from build123d import *

# Parameters (mm, degrees)
SKETCH11_R                        = 5.5626
BASE_FLANGE1_DEPTH                = 2.286
CSK_FOR_M4_FH_MODIFIED_AT_2_COUNT = 2
CSK_FOR_M4_FH_MODIFIED_AT_2_PITCH = 67.76892481
CSK_FOR_M4_FH_MODIFIED_AT_3_COUNT = 2
CSK_FOR_M4_FH_MODIFIED_AT_3_PITCH = 86
CSK_FOR_M4_FH_MODIFIED_AT_4_COUNT = 2
CSK_FOR_M4_FH_MODIFIED_AT_4_PITCH = 52.946886878
CUT_EXTRUDE1_DEPTH                = 82.450069543
FILLET1_R                         = 6.35


# Sheet-metal steps are written as plain solids
with BuildPart() as part:
    # Sketch11 → Base-Flange1 (new body)
    with BuildSketch(Plane.XY):
        Polygon((-49.2252, 40.4876), (-49.2252, -40.4876), (37.337994573, -40.4876), (70.6374, 17.188662062), (70.6374, 40.4876), align=None)
        with Locations((57.15, 27.0002)):
            Circle(SKETCH11_R, mode=Mode.SUBTRACT)
    extrude(amount=-BASE_FLANGE1_DEPTH)

    # Sketch15 → CSK for M4 FH Modified (revolve, cut)
    with BuildSketch(Plane(origin=(36.062834422, 23.419478506, -2.286), x_dir=(0, 1, 0), z_dir=(1, 0, 0))):
        Polygon((0, 0), (0, 2.286), (3.175, 2.286), (3.175, 1.524), (4.699, 0), align=None)
    csk_for_m4_fh_modified = revolve(axis=Axis((36.062834422, 23.419478506, -8.636), (0, 0, 1)), mode=Mode.SUBTRACT)

    # CSK for M4 FH Modified at 2: CSK for M4 FH Modified ×2
    with Locations(*[Vector(-0.9961946980917455, 0.08715574274765803, 0) * (i * CSK_FOR_M4_FH_MODIFIED_AT_2_PITCH) for i in range(1, CSK_FOR_M4_FH_MODIFIED_AT_2_COUNT)]):
        add(csk_for_m4_fh_modified, mode=Mode.SUBTRACT)

    # CSK for M4 FH Modified at 3: CSK for M4 FH Modified ×2
    with Locations(*[Vector(-0.838670567945423, -0.5446390350150286, 0) * (i * CSK_FOR_M4_FH_MODIFIED_AT_3_PITCH) for i in range(1, CSK_FOR_M4_FH_MODIFIED_AT_3_COUNT)]):
        add(csk_for_m4_fh_modified, mode=Mode.SUBTRACT)

    # CSK for M4 FH Modified at 4: CSK for M4 FH Modified ×2
    with Locations(*[Vector(-0.08715574274765796, -0.9961946980917455, 0) * (i * CSK_FOR_M4_FH_MODIFIED_AT_4_PITCH) for i in range(1, CSK_FOR_M4_FH_MODIFIED_AT_4_COUNT)]):
        add(csk_for_m4_fh_modified, mode=Mode.SUBTRACT)

    # Sketch17 → Cut-Extrude1 (cut, through all)
    with BuildSketch(Plane.XY):
        Polygon((-34.546735645, 48.1076), (-56.8452, 0.288388874), (-56.8452, 48.1076), align=None)
    extrude(amount=-CUT_EXTRUDE1_DEPTH, mode=Mode.SUBTRACT)

    # Fillet1
    fillet1_edges = [part.edges().sort_by_distance(p)[0] for p in [
        (-49.2252, 16.629531608, -1.143),
        (-38.1, 40.4876, -1.143),
        (37.337994573, -40.4876, -1.143),
        (-49.2252, -40.4876, -1.143),
        (70.6374, 40.4876, -1.143),
    ]]
    fillet(fillet1_edges, radius=FILLET1_R)


solid = part.part
Work out the finished part from the listing and answer in its coordinate system (mm). Round coordinates to 2 decimals unless told otherwise and drop trailing zeros. Loops run counter-clockwise (first coordinate to the right, second up) from the corner with the lowest first, then second, coordinate; pieces in that order, holes last. Notation, with made-up numbers: M 42,60.5 L 71,60.5 A7 ccw 71,68.5 Z; hole C 25,43.5 d11. An arc over 180 degrees is marked long. One line per question, with ' | ' between items. Start each with the question number.
(1) A cutting plane is placed at B-B on z = -1.75. Write down the section's boundary in (x, y), plus the area to 3 significant figures.
(2) A cutting plane is placed at A-A on x = 57.15. Write down the section's boundary in (y, z).
(3) For a pull along X with two mould halves and no side action, classify faces 1 (the face through (54.684, -10.443, -1.127)), 2 (the face through (-33.25, -21.95, -0.39)), 3 (the face through (-37.509, 39.466, -1.127)), 4 (the face through (62.3, 24.9, -1.1)) as released by +X, released by -X, zero draft, split by the parting line, or undercut.
(4) Find the intervals of material crossed by line 1 (Y direction, x = 34.5, z = -1.5); line 2 (Y direction, x = 33, z = -1.85); line 3 (X direction, y = 27, z = -0.6), in increasing order.
(5) Flat-ended cylindrical pins translate along their axes: pin 1 Ø5 at (x, y) = (31.45, -29.33) entering from -Z; pin 2 Ø8.5 at (x, y) = (-36.06, -23.42) entering from -Z. Find the tip coordinate at first contact, or state that the pin passes through.
(6) A cutting plane is placed at D-D on y = -17. Write down the section's boundary in (x, z).
(7) A cutting plane is placed at C-C on y = 4.5. Write down the section's boundary in (x, z), plus the area to 3 significant figures.
Geometry check:
1) outline: M -49.23,-34.14 A6.35 ccw -42.88,-40.49 L 33.67,-40.49 A6.35 ccw 39.17,-37.31 L 70.64,17.19 L 70.64,34.14 A6.35 ccw 64.29,40.49 L -34.05,40.49 A6.35 ccw -39.81,36.82 L -48.63,17.91 A6.35 ccw -49.23,15.22 Z; hole C -36.06,-23.42 d8.33; hole C -31.45,29.33 d8.33; hole C 31.45,-29.33 d8.33; hole C 36.06,23.42 d8.33; hole C 57.15,27 d11.13 | area: 8,280 mm²
2) outline: M -6.17,-2.29 L 21.44,-2.29 L 21.44,0 L -6.17,0 Z; M 32.56,-2.29 L 40.49,-2.29 L 40.49,0 L 32.56,0 Z
3) face 1: released by +X | face 2: undercut | face 3: released by -X | face 4: undercut
4) line 1: y = -40.43 to -31.78, -26.88 to 19.83, 27.01 to 40.49 | line 2: y = -40.49 to -33.3, -25.36 to 20.45, 26.38 to 40.49 | line 3: x = -44.39 to -33.61, -29.29 to 51.59, 62.71 to 70.64
5) pin 1: passes through | pin 2: stops at z = -1.84
6) outline: M -49.23,-2.29 L 50.9,-2.29 L 50.9,0 L -49.23,0 Z
7) outline: M -49.23,-2.29 L 63.31,-2.29 L 63.31,0 L -49.23,0 Z | area: 257 mm²
